Check sheet for the drawn part. Datum: minimum x, y, z corner. Units: mm. Give positions to 0.01 mm unless a question says otherwise; leave off trailing zeros. Order: outer loops, then holes, each group sorted by start corner. A loop starts at its lowest first (then second) coordinate and runs counter-clockwise, first axis right, second up.
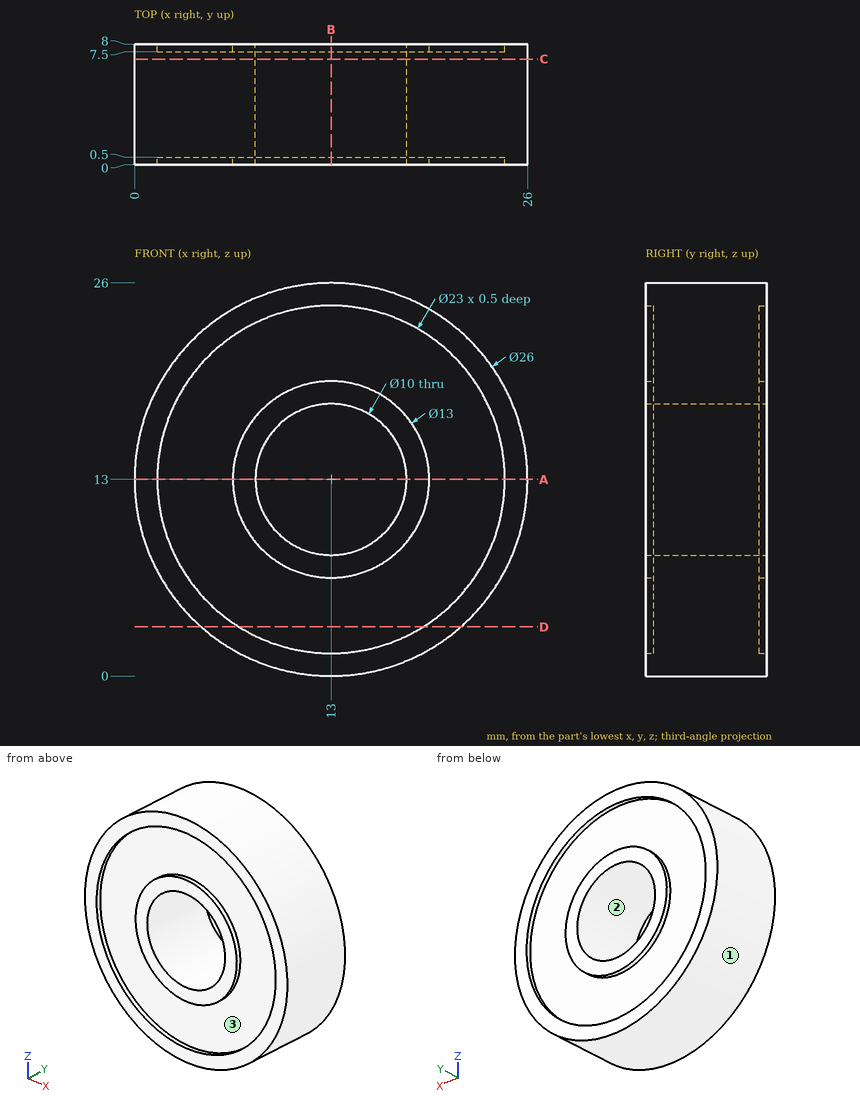
Item 1: Sectioned sample at B-B (x = 13). Enter the section's corners in (y, z), and give its area (3 significant figures).
Reported:
outline: (0, 0) - (8, 0) - (8, 1.5) - (7.5, 1.5) - (7.5, 6.5) - (8, 6.5) - (8, 8) - (0, 8) - (0, 6.5) - (0.5, 6.5) - (0.5, 1.5) - (0, 1.5) - close; (0, 18) - (8, 18) - (8, 19.5) - (7.5, 19.5) - (7.5, 24.5) - (8, 24.5) - (8, 26) - (0, 26) - (0, 24.5) - (0.5, 24.5) - (0.5, 19.5) - (0, 19.5) - close
area: 118 mm2
Item 2: Gauge pin test, flat ends, axial feed: pin 1 (1 mm diameter, centred on y = 1.5, z = 22.5, fed in from +X); pin 2 (3 mm diameter, centred on x = 8, y = 3.5, fed in from -Z); pin 3 (3 mm diameter, centred on x = 15, y = 2.5, fed in from -Z). Record the tip position at first contact, or that the pin passes through.
Reported:
pin 1: stops at x = 22.38
pin 2: stops at z = 0.48
pin 3: stops at z = 0.01
Item 3: Draft check along X on the marked faces 1, 2 and 3. Enter one of: released by +X, released by -X, zero draft, split by the parting line, or undercut.
Reported:
face 1: split by the parting line
face 2: undercut
face 3: undercut
Item 4: Sectioned sample at D-D (z = 3.25). Enter the section's corners in (x, y), and give its area (3 significant figures).
Reported:
outline: (4.4, 0) - (6.9, 0) - (6.9, 0.5) - (19.1, 0.5) - (19.1, 0) - (21.6, 0) - (21.6, 8) - (19.1, 8) - (19.1, 7.5) - (6.9, 7.5) - (6.9, 8) - (4.4, 8) - close
area: 125 mm2
Item 5: Scan lines: L1, parallel to X at y = 0.1, z = 13; L2, parallel to Z at x = 12.75, y = 1.75; L3, parallel to Y at x = 2.25, z = 10. Record each from-to range of solid material in increasing order.
Reported:
L1: x = 0 to 1.5, 6.5 to 8, 18 to 19.5, 24.5 to 26
L2: z = 0 to 8.01, 17.99 to 26
L3: y = 0.5 to 7.5
Item 6: Sectioned sample at A-A (z = 13). Enter the section's corners in (x, y), and give its area (3 significant figures).
Reported:
outline: (0, 0) - (1.5, 0) - (1.5, 0.5) - (6.5, 0.5) - (6.5, 0) - (8, 0) - (8, 8) - (6.5, 8) - (6.5, 7.5) - (1.5, 7.5) - (1.5, 8) - (0, 8) - close; (18, 0) - (19.5, 0) - (19.5, 0.5) - (24.5, 0.5) - (24.5, 0) - (26, 0) - (26, 8) - (24.5, 8) - (24.5, 7.5) - (19.5, 7.5) - (19.5, 8) - (18, 8) - close
area: 118 mm2
Item 7: Sectioned sample at C-C (y = 7). Enter the section's corners in (x, z), and give its area (3 significant figures).
Reported:
outline: circle Ø26 at (13, 13); hole circle Ø10 at (13, 13)
area: 452 mm2
